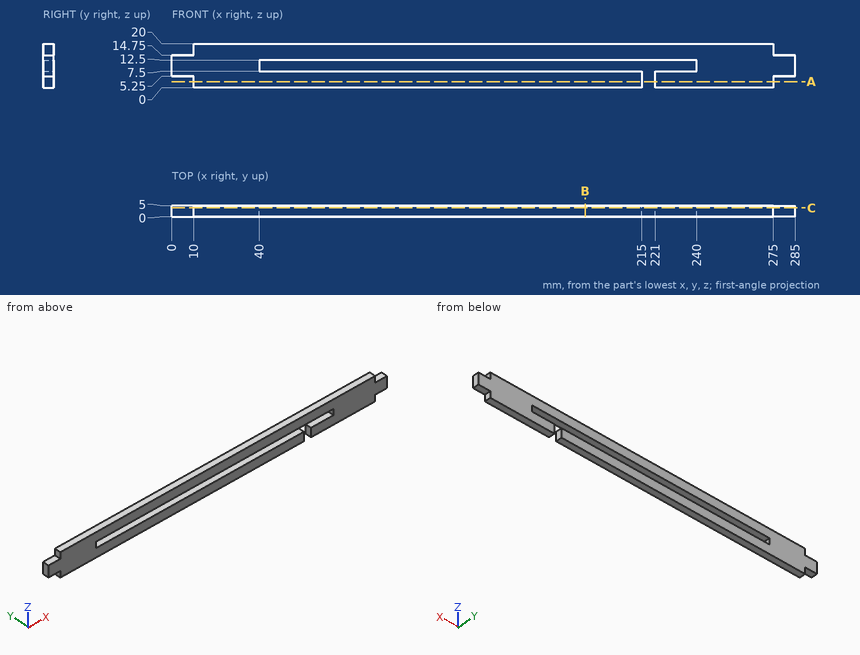
The figure shows three views and two pictorial views of one solid part (mm, origin at its lowest corner). Answer the questions. Coordinates: 2 decimals unless noted, no trailing zeros. Loops run counter-clockwise (first coordinate to the right, second up) from the corner with the lowest first, then second, coordinate; pieces in that order, holes last. Notation, with made-up numbers: M -17,81 L 6,81 A26 cw 6,118 Z; hole C 55.5,17.25 d8. An arc over 180 degrees is marked long. Answer as CSV lines item,"result". Start each with the question number.
(1) The part is cut by section B-B (x = 189). Give the vertices of the cut face in (y, z).
(2) Given pin 1 (2.5 mm diameter, centred on y = 2.5, z = 3.5, fed in from +X); pin 2 (1.5 mm diameter, centred on x = 282.5, y = 3.5, fed in from +Z); pin 3 (2.5 mm diameter, centred on y = 2, z = 16.5, fed in from -X), each flat-ended and moving along its own axis, determine where each tip first touches the part or whether it passes through.
(3) The part is cut by section C-C (y = 4). Give the vertices of the cut face in (x, z), and give its area (4 significant figures).
(4) Find the intervals of material crossed by L1, parallel to X at y = 3.4, z = 9.25; L2, parallel to Z at x = 170.5, y = 2.35; L3, parallel to X at y = 4, z = 2, in increasing order. Write a range as [from, to].
(5) The part is cut by section A-A (z = 2.75). Give the vertices of the cut face in (x, y), and give its area (4 significant figures).
Determined:
1,outline,"M 0,0 L 5,0 L 5,7.5 L 0,7.5 Z; M 0,12.5 L 5,12.5 L 5,20 L 0,20 Z"
2,pin 1,"x = 275"
2,pin 2,"z = 14.75"
2,pin 3,"x = 10"
3,outline,"M 0,5.25 L 10,5.25 L 10,0 L 215,0 L 215,7.5 L 40,7.5 L 40,12.5 L 240,12.5 L 240,7.5 L 221,7.5 L 221,0 L 275,0 L 275,5.25 L 285,5.25 L 285,14.75 L 275,14.75 L 275,20 L 10,20 L 10,14.75 L 0,14.75 Z"
3,area,"4,445 mm2"
4,L1,"[0, 40], [240, 285]"
4,L2,"[0, 7.5], [12.5, 20]"
4,L3,"[10, 215], [221, 275]"
5,outline,"M 10,0 L 215,0 L 215,5 L 10,5 Z; M 221,0 L 275,0 L 275,5 L 221,5 Z"
5,area,"1,295 mm2"
